Can you work these out from the model? Positions are in its coordinate system, mm. Face numbers are marked on the shaded views. A direction names the side the tool comes from. Give positions to 0.01 mm unless a question says otherwise; leave off trailing zeros. Order: outer loops, then holes, each group sorted by start corner. A loop starts at its lowest first (then second) coordinate and runs counter-clockwise, first axis right, second up. Notation, with made-up numbers: M 82,20 L 94,20 A35 ccw 94,58 Z; hole C 49.25,-40 d8. An arc over 180 degrees is marked long. Use one line per item in the form item = value. Start each with the question number.
1. For the marked faces 1, 2 and 3, which set-ups out of +Z, -Z, +X, -X, +Y, -Y let a thin tool reach every point of the face, with its end or its side?
2. I want a section at B-B, the plane x = -11.75. List the corners of the cut face in (y, z) for me, and give its area (3 significant figures).
3. I need wall thicknesses on L1, parallel to Y at x = -7.5, z = 4; L2, parallel to Z at x = -10.75, y = 4; L3, parallel to Z at x = -14, y = 10. Which ranges of each line are inside material? Lowest first, please.
4. I want a section at A-A, the plane y = 5.5. Count the separate pieces of the cut face and the enclosed holes in it, and give its area (3 significant figures).
5. I want a section at C-C, the plane z = 30. List the corners of the cut face in (x, y) for me.
6. I want a section at D-D, the plane x = -4. List the corners of the cut face in (y, z) for me.
7. We'd pull the mould along Z, two halves only. Please class the marked faces 4, 5, 6 and 7: +Z half, -Z half, draft (parallel to the pull), parting line (faces both ways), or undercut.
8. Will these pins go through, and if not, where does the flat tip stop? P1, Ø2.5, axis at x = -4, z = 20, coming from the -Y side; P2, Ø3, axis at y = 6, z = 18, coming from the -X side; P3, Ø4, axis at y = 6.5, z = 19.5, coming from the +X side (3 decimals); P4, Ø3, axis at y = 5.5, z = 30, coming from the -X side.
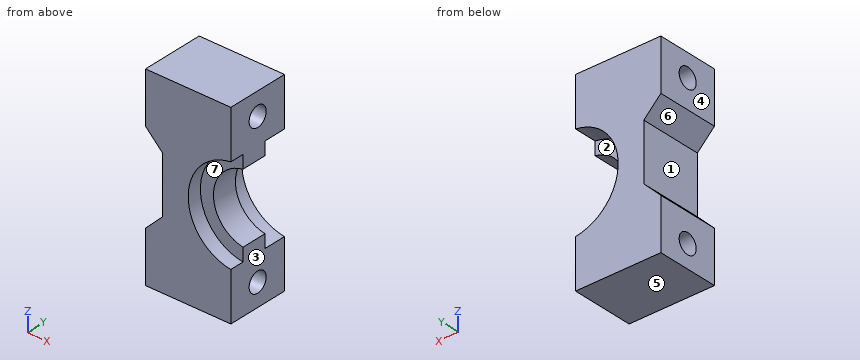
```python
from build123d import *

# Parameters (mm, degrees)
SKETCH2_W           = 34
SKETCH2_H           = 11
SKETCH2_R           = 1.75
BOSS_EXTRUDE1_DEPTH = 16
SKETCH5_W           = 1
SKETCH5_H           = 34
SKETCH5_W_2         = 3
SKETCH5_H_2         = 10
CUT_EXTRUDE1_DEPTH  = 40.153543901
CHAMFER1_SIZE       = 3


with BuildPart() as part:
    # Sketch2 → Boss-Extrude1 (new body)
    with BuildSketch(Plane(origin=(0, 0, 0), x_dir=(0, 0, -1), z_dir=(1, 0, 0))):
        with Locations((-17, 5.5)):
            Rectangle(SKETCH2_W, SKETCH2_H)
        with Locations((-30, 5.5)):
            Circle(SKETCH2_R, mode=Mode.SUBTRACT)
        with Locations((-4, 5.5)):
            Circle(SKETCH2_R, mode=Mode.SUBTRACT)
    extrude(amount=-BOSS_EXTRUDE1_DEPTH)

    # Sketch4 → Cut-Revolve1 (revolve, cut)
    with BuildSketch(Plane(origin=(0, 0, 0), x_dir=(0, 0, -1), z_dir=(1, 0, 0))):
        Polygon((-17, 0), (-25.5, 0), (-25.5, 2.5), (-23.2, 2.5), (-23.2, 7), (-25.5, 7), (-25.5, 11), (-17, 11), align=None)
    revolve(axis=Axis((0, 0, 17), (0, 1, 0)), mode=Mode.SUBTRACT)

    # Sketch5 → Cut-Extrude1 (cut, through all)
    with BuildSketch(Plane(origin=(0, 11, 0), x_dir=(1, 0, 0), z_dir=(0, 1, 0))):
        with Locations((-0.5, -17)):
            Rectangle(SKETCH5_W, SKETCH5_H)
        with Locations((-14.5, -17)):
            Rectangle(SKETCH5_W_2, SKETCH5_H_2)
    extrude(amount=-CUT_EXTRUDE1_DEPTH, mode=Mode.SUBTRACT)

    # Chamfer1
    chamfer1_edges = [part.edges().sort_by_distance(p)[0] for p in [
        (-16, 5.5, 22),
        (-16, 5.5, 12),
    ]]
    chamfer(chamfer1_edges, length=CHAMFER1_SIZE - 0.0001)  # a hair under: the kernel refuses the full size


solid = part.part
```
Check result:
q1.face_1 = -X, +Y, -Y
q1.face_2 = +X, +Y
q1.face_3 = +Z, -Z, +X, +Y, -Y
q2.outline = M 0,0 L 11,0 L 11,34 L 0,34 Z; hole C 5.5,4 d3.5; hole C 5.5,30 d3.5
q2.area = 355 mm2
q3.L1 = 0 to 3.75, 7.25 to 11
q3.L2 = 0 to 3.1, 4.9 to 29.1, 30.9 to 34
q3.L3 = 0 to 11, 23 to 34
q4.separate_pieces = 3
q4.enclosed_holes = 0
q4.area = 318 mm2
q5.outline = M -16,0 L -1,0 L -1,3.75 L -16,3.75 Z; M -16,7.25 L -1,7.25 L -1,11 L -16,11 Z
q6.outline = M 0,0 L 11,0 L 11,9.5 L 7,9.5 L 7,12.26 L 2.5,12.26 L 2.5,9.5 L 0,9.5 Z; M 0,24.5 L 2.5,24.5 L 2.5,21.74 L 7,21.74 L 7,24.5 L 11,24.5 L 11,34 L 0,34 Z; hole C 5.5,4 d3.5; hole C 5.5,30 d3.5
q7.face_4 = draft
q7.face_5 = -Z half
q7.face_6 = undercut
q7.face_7 = undercut
q8.P1 = 2.5
q8.P2 = -13
q8.P3 = -4.265
q8.P4 = through
